Geometry: see drawing. Coordinates: mm, zero at the bounding-box minimum. A direction names the side the tool comes from. Coordinates: 2 decimals unless noted, no trailing zeros. Write each loop counter-clockwise with the first axis right and the second up, starting at its lowest first coordinate (ties: lowest second). Pieces come first, ordered by that corner, then holes.
1) Section query D-D (x = 4). Output: boundary loops of the cut face in (y, z), then the cut area to 3 significant figures.
2) Section query C-C (x = 11.5). Output: boundary loops of the cut face in (y, z).
3) Set-up query: the marked faces 1 and 2. Return all of +Z, -Z, +X, -X, +Y, -Y with unobstructed straight access to the full face (end or side cutting, diameter ignored); none if empty.
4) Pin query (flat end, axial travel): pin 1 Ø5 at (x, z) = (11.5, 4.5) entering from +Y; pin 2 Ø4 at (x, z) = (8.5, 2) entering from +Y; pin 3 Ø2 at (x, z) = (25, 8.5) entering from -Y; pin 4 Ø2.5 at (y, z) = (6, 8.5) entering from -X. Return the tip coordinate at first contact, or that it passes through.
5) Line query: L1, parallel to X at y = 11.75, z = 6.75; L2, parallel to X at y = 2.25, z = 4.5; L3, parallel to Z at x = 6.5, y = 4. Output: solid intervals per line, ascending.
6) Section query A-A (z = 7). Output: boundary loops of the cut face in (x, y).
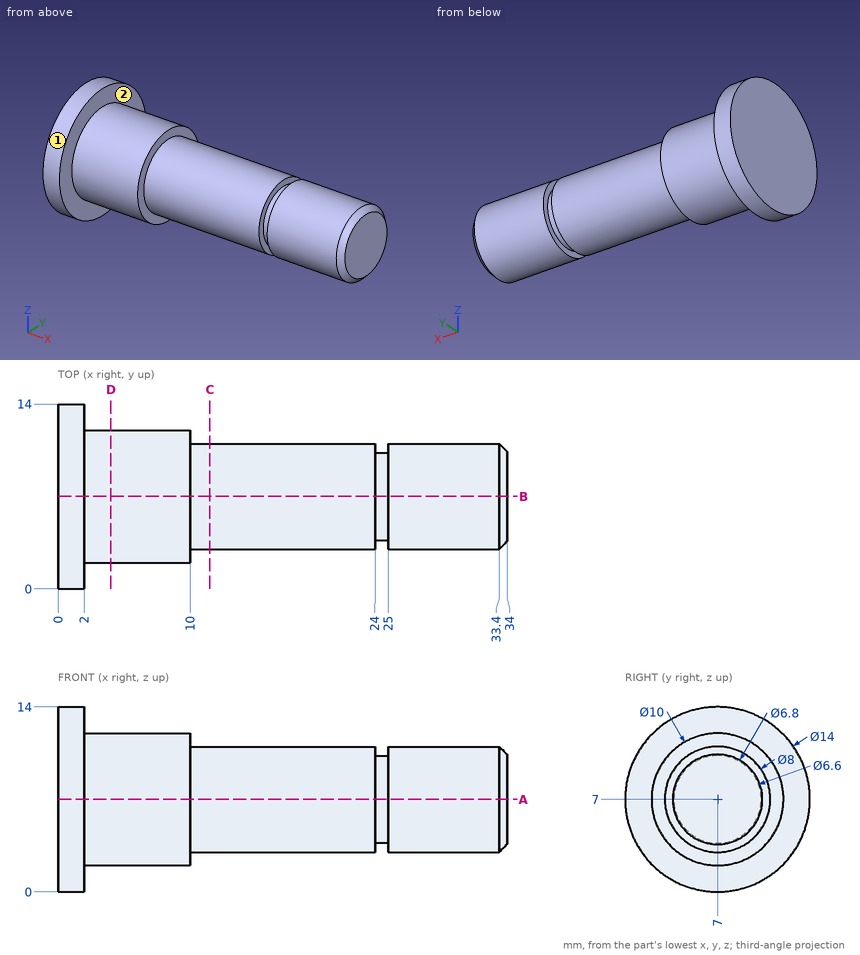
Answer:
1. outline: circle Ø10 at (7, 7)
1. area: 78.5 mm2
2. outline: circle Ø8 at (7, 7)
3. face 1: +X, -X
3. face 2: +X
4. pin 1: stops at y = 11.97
4. pin 2: stops at y = 11
4. pin 3: stops at y = 3.03
4. pin 4: stops at x = 0
5. L1: x = 0 to 10
5. L2: x = 0 to 2
5. L3: z = 3 to 11
6. outline: (0, 0) - (2, 0) - (2, 2) - (10, 2) - (10, 3) - (24, 3) - (24, 3.7) - (25, 3.7) - (25, 3) - (33.4, 3) - (34, 3.6) - (34, 10.4) - (33.4, 11) - (25, 11) - (25, 10.3) - (24, 10.3) - (24, 11) - (10, 11) - (10, 12) - (2, 12) - (2, 14) - (0, 14) - close
